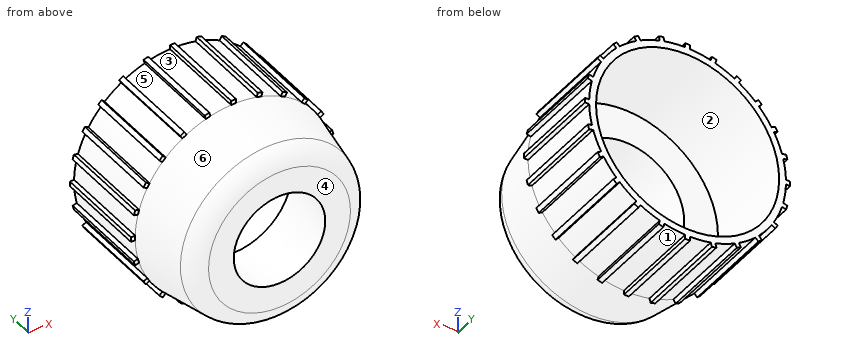
from build123d import *

# Parameters (mm, degrees)
BOSS_EXTRUDE1_DEPTH = 20


with BuildPart() as part:
    # Sketch1 → Revolve1 (revolve)
    with BuildSketch(Plane.XY, mode=Mode.PRIVATE) as revolve1_sk:
        with BuildLine():
            Line((12.644904711, 15), (10, 0))
            Line((10, 0), (15.498696765, 0))
            ThreePointArc((15.498696765, 0), (18.069847203, 0.935822228), (19.437927777, 3.305407289))
            Line((19.437927777, 3.305407289), (21.5, 15))
            Line((21.5, 15), (21.5, 35))
            Line((21.5, 35), (20, 35))
            Line((20, 35), (20, 15))
            Line((20, 15), (12.644904711, 15))
        make_face()
    revolve(revolve1_sk.sketch.rotate(Axis((0, 0, 0), (0, 1, 0)), 90), axis=Axis((0, 0, 0), (0, 1, 0)))

    # Sketch2 → Boss-Extrude1 (add)
    with BuildSketch(Plane(origin=(0, 35, 0), x_dir=(1, 0, 0), z_dir=(0, 1, 0))):
        with BuildLine():
            Line((21.49358916, -0.525), (22.42, -0.525))
            Line((22.42, -0.525), (22.42, 0.525))
            Line((22.42, 0.525), (21.49358916, 0.525))
            ThreePointArc((21.49358916, 0.525), (21.5, 0), (21.49358916, -0.525))
        make_face()
        with BuildLine():
            Line((20.625332871, -6.070061281), (21.520177027, -6.30983405))
            Line((21.520177027, -6.30983405), (21.791937024, -5.295611932))
            Line((21.791937024, -5.295611932), (20.897092868, -5.055839164))
            ThreePointArc((20.897092868, -5.055839164), (20.767405265, -5.56460947), (20.625332871, -6.070061281))
        make_face()
        with BuildLine():
            Line((18.351494231, -11.201457917), (19.153789553, -11.664663337))
            Line((19.153789553, -11.664663337), (19.678789553, -10.755336663))
            Line((19.678789553, -10.755336663), (18.876494231, -10.292131243))
            ThreePointArc((18.876494231, -10.292131243), (18.619546181, -10.75), (18.351494231, -11.201457917))
        make_face()
        with BuildLine():
            Line((14.827031587, -15.569493708), (15.482102974, -16.224565094))
            Line((15.482102974, -16.224565094), (16.224565094, -15.482102974))
            Line((16.224565094, -15.482102974), (15.569493708, -14.827031587))
            ThreePointArc((15.569493708, -14.827031587), (15.202795796, -15.202795796), (14.827031587, -15.569493708))
        make_face()
        with BuildLine():
            Line((10.292131243, -18.876494231), (10.755336663, -19.678789553))
            Line((10.755336663, -19.678789553), (11.664663337, -19.153789553))
            Line((11.664663337, -19.153789553), (11.201457917, -18.351494231))
            ThreePointArc((11.201457917, -18.351494231), (10.75, -18.619546181), (10.292131243, -18.876494231))
        make_face()
        with BuildLine():
            Line((5.055839164, -20.897092868), (5.295611932, -21.791937024))
            Line((5.295611932, -21.791937024), (6.30983405, -21.520177027))
            Line((6.30983405, -21.520177027), (6.070061281, -20.625332871))
            ThreePointArc((6.070061281, -20.625332871), (5.56460947, -20.767405265), (5.055839164, -20.897092868))
        make_face()
        with BuildLine():
            Line((-0.525, -21.49358916), (-0.525, -22.42))
            Line((-0.525, -22.42), (0.525, -22.42))
            Line((0.525, -22.42), (0.525, -21.49358916))
            ThreePointArc((0.525, -21.49358916), (0, -21.5), (-0.525, -21.49358916))
        make_face()
        with BuildLine():
            Line((-6.070061281, -20.625332871), (-6.30983405, -21.520177027))
            Line((-6.30983405, -21.520177027), (-5.295611932, -21.791937024))
            Line((-5.295611932, -21.791937024), (-5.055839164, -20.897092868))
            ThreePointArc((-5.055839164, -20.897092868), (-5.56460947, -20.767405265), (-6.070061281, -20.625332871))
        make_face()
        with BuildLine():
            Line((-11.201457917, -18.351494231), (-11.664663337, -19.153789553))
            Line((-11.664663337, -19.153789553), (-10.755336663, -19.678789553))
            Line((-10.755336663, -19.678789553), (-10.292131243, -18.876494231))
            ThreePointArc((-10.292131243, -18.876494231), (-10.75, -18.619546181), (-11.201457917, -18.351494231))
        make_face()
        with BuildLine():
            Line((-15.569493708, -14.827031587), (-16.224565094, -15.482102974))
            Line((-16.224565094, -15.482102974), (-15.482102974, -16.224565094))
            Line((-15.482102974, -16.224565094), (-14.827031587, -15.569493708))
            ThreePointArc((-14.827031587, -15.569493708), (-15.202795796, -15.202795796), (-15.569493708, -14.827031587))
        make_face()
        with BuildLine():
            Line((-18.876494231, -10.292131243), (-19.678789553, -10.755336663))
            Line((-19.678789553, -10.755336663), (-19.153789553, -11.664663337))
            Line((-19.153789553, -11.664663337), (-18.351494231, -11.201457917))
            ThreePointArc((-18.351494231, -11.201457917), (-18.619546181, -10.75), (-18.876494231, -10.292131243))
        make_face()
        with BuildLine():
            Line((-20.897092868, -5.055839164), (-21.791937024, -5.295611932))
            Line((-21.791937024, -5.295611932), (-21.520177027, -6.30983405))
            Line((-21.520177027, -6.30983405), (-20.625332871, -6.070061281))
            ThreePointArc((-20.625332871, -6.070061281), (-20.767405265, -5.56460947), (-20.897092868, -5.055839164))
        make_face()
        with BuildLine():
            Line((-21.49358916, 0.525), (-22.42, 0.525))
            Line((-22.42, 0.525), (-22.42, -0.525))
            Line((-22.42, -0.525), (-21.49358916, -0.525))
            ThreePointArc((-21.49358916, -0.525), (-21.5, 0), (-21.49358916, 0.525))
        make_face()
        with BuildLine():
            Line((-20.625332871, 6.070061281), (-21.520177027, 6.30983405))
            Line((-21.520177027, 6.30983405), (-21.791937024, 5.295611932))
            Line((-21.791937024, 5.295611932), (-20.897092868, 5.055839164))
            ThreePointArc((-20.897092868, 5.055839164), (-20.767405265, 5.56460947), (-20.625332871, 6.070061281))
        make_face()
        with BuildLine():
            Line((-18.351494231, 11.201457917), (-19.153789553, 11.664663337))
            Line((-19.153789553, 11.664663337), (-19.678789553, 10.755336663))
            Line((-19.678789553, 10.755336663), (-18.876494231, 10.292131243))
            ThreePointArc((-18.876494231, 10.292131243), (-18.619546181, 10.75), (-18.351494231, 11.201457917))
        make_face()
        with BuildLine():
            Line((-14.827031587, 15.569493708), (-15.482102974, 16.224565094))
            Line((-15.482102974, 16.224565094), (-16.224565094, 15.482102974))
            Line((-16.224565094, 15.482102974), (-15.569493708, 14.827031587))
            ThreePointArc((-15.569493708, 14.827031587), (-15.202795796, 15.202795796), (-14.827031587, 15.569493708))
        make_face()
        with BuildLine():
            Line((-10.292131243, 18.876494231), (-10.755336663, 19.678789553))
            Line((-10.755336663, 19.678789553), (-11.664663337, 19.153789553))
            Line((-11.664663337, 19.153789553), (-11.201457917, 18.351494231))
            ThreePointArc((-11.201457917, 18.351494231), (-10.75, 18.619546181), (-10.292131243, 18.876494231))
        make_face()
        with BuildLine():
            Line((-5.055839164, 20.897092868), (-5.295611932, 21.791937024))
            Line((-5.295611932, 21.791937024), (-6.30983405, 21.520177027))
            Line((-6.30983405, 21.520177027), (-6.070061281, 20.625332871))
            ThreePointArc((-6.070061281, 20.625332871), (-5.56460947, 20.767405265), (-5.055839164, 20.897092868))
        make_face()
        with BuildLine():
            Line((0.525, 21.49358916), (0.525, 22.42))
            Line((0.525, 22.42), (-0.525, 22.42))
            Line((-0.525, 22.42), (-0.525, 21.49358916))
            ThreePointArc((-0.525, 21.49358916), (0, 21.5), (0.525, 21.49358916))
        make_face()
        with BuildLine():
            Line((6.070061281, 20.625332871), (6.30983405, 21.520177027))
            Line((6.30983405, 21.520177027), (5.295611932, 21.791937024))
            Line((5.295611932, 21.791937024), (5.055839164, 20.897092868))
            ThreePointArc((5.055839164, 20.897092868), (5.56460947, 20.767405265), (6.070061281, 20.625332871))
        make_face()
        with BuildLine():
            Line((11.201457917, 18.351494231), (11.664663337, 19.153789553))
            Line((11.664663337, 19.153789553), (10.755336663, 19.678789553))
            Line((10.755336663, 19.678789553), (10.292131243, 18.876494231))
            ThreePointArc((10.292131243, 18.876494231), (10.75, 18.619546181), (11.201457917, 18.351494231))
        make_face()
        with BuildLine():
            Line((15.569493708, 14.827031587), (16.224565094, 15.482102974))
            Line((16.224565094, 15.482102974), (15.482102974, 16.224565094))
            Line((15.482102974, 16.224565094), (14.827031587, 15.569493708))
            ThreePointArc((14.827031587, 15.569493708), (15.202795796, 15.202795796), (15.569493708, 14.827031587))
        make_face()
        with BuildLine():
            Line((18.876494231, 10.292131243), (19.678789553, 10.755336663))
            Line((19.678789553, 10.755336663), (19.153789553, 11.664663337))
            Line((19.153789553, 11.664663337), (18.351494231, 11.201457917))
            ThreePointArc((18.351494231, 11.201457917), (18.619546181, 10.75), (18.876494231, 10.292131243))
        make_face()
        with BuildLine():
            Line((20.897092868, 5.055839164), (21.791937024, 5.295611932))
            Line((21.791937024, 5.295611932), (21.520177027, 6.30983405))
            Line((21.520177027, 6.30983405), (20.625332871, 6.070061281))
            ThreePointArc((20.625332871, 6.070061281), (20.767405265, 5.56460947), (20.897092868, 5.055839164))
        make_face()
    extrude(amount=-BOSS_EXTRUDE1_DEPTH)


solid = part.part
For this review, take the finished solid that the model builds, in its own axes (mm). Face numbers are marked on the shaded views. A direction names the side the tool comes from. Give positions to 0.01 mm unless a question says otherwise; leave off trailing zeros. Loops run counter-clockwise (first coordinate to the right, second up) from the corner with the lowest first, then second, coordinate; pieces in that order, holes last. Notation, with made-up numbers: M 72.5,-18 L 122.5,-18 A12 ccw 122.5,-7 Z; hole C -23.75,-23.75 d10. An arc over 180 degrees is marked long. Answer as a JSON object with one key per item and string values. Group by question number.
Q1. Mouldability with a two-part tool opening along X and no side actions: class the marked faces 4, 5 and 6 as +X half, -X half, draft (parallel to the pull), parting line (faces both ways), or undercut.
Q2. Tool access review of the marked faces 1, 2 and 3: name each direction out of +Z, -Z, +X, -X, +Y, -Y from which nothing blocks a thin tool from reaching the whole face with its end or side.
Q3. Insertion check: P1, Ø8, axis at x = 17, y = 11.5, coming from the -Z side; P2, Ø0.5, axis at x = 22, z = 0, coming from the -Y side; P3, Ø8, axis at y = 21, z = 6.5, coming from the +X side. Each pin has a flat end and moves straight along its axis. Give the tip position at first contact, or say it passes through.
Q4. Add section B-B on y = 12.5. Give the boundary of the cut face in (x, z).
Q5. For probe 1 along X at (y, z) = (28, 0); probe 2 along X at (y, z) = (21, -18); probe 3 along Z at (x, y) = (-5, 22), list the stretches that pass through material, from the lowest coordinate up. Write a range as [from, to].
Q6. Add section A-A on y = 9. Give the boundary of the cut face in (x, z).
Checked values:
{
 "1": {"face 4": "draft", "face 5": "undercut", "face 6": "parting line"},
 "2": {"face 1": "-Z, +Y, -Y", "face 2": "+Y", "face 3": "+Z, +Y, -Y"},
 "3": {"P1": "z = -16.47", "P2": "y = 15", "P3": "x = 21.79"},
 "4": {"outline": "C 0,0 d42.12; hole C 0,0 d24.41"},
 "5": {"probe 1": "[-22.42, -20], [20, 22.42]", "probe 2": "[-11.76, -8.72], [8.72, 11.76]", "probe 3": "[-20.91, -19.36], [19.36, 20.91]"},
 "6": {"outline": "C 0,0 d40.88; hole C 0,0 d23.17"}
}
